Check sheet for the modelled part. Datum: model origin and axes. Units: mm. A direction names the side the tool comes from. Give positions to 0.01 mm unless a question says otherwise; leave off trailing zeros. Write each loop counter-clockwise with the first axis right and the second up, starting at its lowest first coordinate (ties: lowest second). Pieces come first, ordered by that corner, then holes. Notation, with made-up numbers: M -17.5,19 L 35.5,19 A21 cw 35.5,28 Z; hole C 80.5,48 d4. An arc over 180 degrees is marked long. Write item = value, one per line. Start each with the question number.
1) Scan lines: L1, parallel to Y at x = 12, z = 0; L2, parallel to Y at x = 28.5, z = 0.5; L3, parallel to X at y = -31, z = -19. Record each from-to range of solid material in increasing order.
2) Sectioned sample at B-B, the plane x = 37. Record the cut outline in (y, z).
3) Set-up check for faces 1 (the face through (15.5, 24.2, 24.2)), 2 (the face through (33.05, 26.36, -5.85)), 3 (the face through (20, 0, 22.25)): record each of +Z, -Z, +X, -X, +Y, -Y from which the full face is reachable in a straight line by a thin tool's end or side.
4) Sectioned sample at D-D, the plane x = 9. Record the cut outline in (y, z).
5) Gauge pin test, flat ends, axial feed: pin 1 (4 mm diameter, centred on x = 10.5, y = -10.5, fed in from -Z); pin 2 (1.5 mm diameter, centred on x = 26.5, y = 12, fed in from +Z); pin 3 (1.5 mm diameter, centred on x = 9, z = -17.5, fed in from +Y). Record the tip position at first contact, or that the pin passes through.
6) Draft check along Y on faces 4 (the face through (0.12, 35.75, -7.94)), 5 (the face through (10, 24.2, -24.2)), 6 (the face through (20, 5, 20)). Enter one of: pulls with the +Y half, pulls with the -Y half, needs draft (parallel to the pull), parting line crosses it, or undercut.
from build123d import *

# Parameters (mm, degrees)
F2_SIZE  = 2.5
F3_W     = 10
F3_H     = 9
F4_DEPTH = 40.001
F5_R     = 1


with BuildPart() as f1:
    # F0 (on Front) → F1 (revolve)
    with BuildSketch(Plane.XZ):
        Polygon((10, 39), (0, 39), (0, 19), (40, 19), (40, 27), (25.3, 27), (25.3, 39), (15.5, 39), (15.5, 34), (10, 34), align=None)
    revolve(axis=Axis((29.337285, 0, 0), (1, 0, 0)))

    # F2
    f2_edges = [f1.edges().sort_by_distance(p)[0] for p in [
        (0, 0, -39),
        (10, 0, -39),
        (15.5, 0, -39),
        (25.3, 0, -39),
    ]]
    chamfer(f2_edges, length=F2_SIZE)

    # F3 (on Right) → F4 (cut, through all)
    with BuildSketch(Plane.YZ):
        with Locations((0, 17.75)):
            Rectangle(F3_W, F3_H)
    extrude(amount=F4_DEPTH, mode=Mode.SUBTRACT)

    # F5
    f5_edges = [f1.edges().sort_by_distance(p)[0] for p in [
        (25.3, 0, -27),
    ]]
    fillet(f5_edges, radius=F5_R)


solid = f1.part
Data:
q1.L1 = -34 to -19, 19 to 34
q1.L2 = -27 to -18.99, 18.99 to 27
q1.L3 = 0 to 10, 15.5 to 25.3
q2.outline = C 0,0 d54; hole M -5,18.33 A19 ccw long 5,18.33 L 5,22.25 L -5,22.25 Z
q3.face_1 = none
q3.face_2 = +X
q3.face_3 = +X, -X
q4.outline = C 0,0 d75; hole M -5,18.33 A19 ccw long 5,18.33 L 5,22.25 L -5,22.25 Z
q5.pin_1 = -36.59
q5.pin_2 = 24.54
q5.pin_3 = 34.09
q6.face_4 = parting line crosses it
q6.face_5 = needs draft
q6.face_6 = undercut
